Geometry: final body of the model. Coordinates: model frame, mm. A direction names the side the tool comes from. Give positions to 0.01 mm unless a question says otherwise; leave off trailing zeros. Write each loop counter-clockwise with the first axis right and the second up, starting at its lowest first coordinate (ties: lowest second). Pieces come first, ordered by that corner, then holes. Notation, with made-up numbers: (23.25, -2) - (48.25, -2) arc R18 ccw to (48.25, 21) - close; hole circle Ø4 at (75, 24). An arc over 180 degrees is marked (long way). One line per question, with ' | ' between items. Start each with the question number.
```python
from build123d import *

# Parameters (mm, degrees)
SKETCH1_R           = 13
BOSS_EXTRUDE1_DEPTH = 12.5
CUT_EXTRUDE1_START  = 3
SKETCH2_R           = 16
CUT_EXTRUDE1_DEPTH  = 37.563240514
SKETCH3_R           = 2.5
CUT_EXTRUDE2_DEPTH  = 52.285962992
CUT_EXTRUDE3_START  = 10
SKETCH5_R           = 16.85
SKETCH5_R_2         = 16
CUT_EXTRUDE3_DEPTH  = 1.3
CHAMFER2_SIZE       = 0.5


with BuildPart() as part:
    # Sketch1 → Boss-Extrude1 (new body)
    with BuildSketch(Plane.XY):
        with BuildLine():
            Line((25, -28), (-25, -28))
            Line((-25, -28), (-25, -23))
            Line((-25, -23), (-10.297842021, -23))
            Line((-10.297842021, -23), (-10.297842021, -17.145099875))
            ThreePointArc((-10.297842021, -17.145099875), (0, 20), (10.297842021, -17.145099875))
            Line((10.297842021, -17.145099875), (10.297842021, -23))
            Line((10.297842021, -23), (25, -23))
            Line((25, -23), (25, -28))
        make_face()
        Circle(SKETCH1_R, mode=Mode.SUBTRACT)
    extrude(amount=BOSS_EXTRUDE1_DEPTH)

    # Sketch2 → Cut-Extrude1 (cut, through all)
    with BuildSketch(Plane.XY.offset(CUT_EXTRUDE1_START)):
        Circle(SKETCH2_R)
    extrude(amount=CUT_EXTRUDE1_DEPTH, mode=Mode.SUBTRACT)

    # Sketch3 → Cut-Extrude2 (cut, through all)
    with BuildSketch(Plane(origin=(0, -23, 0), x_dir=(1, 0, 0), z_dir=(0, 1, 0))):
        with Locations(Location((-20, -6.25, 0), (0, 0, 180))):
            Circle(SKETCH3_R)
        with Locations(Location((20, -6.25, 0), (0, 0, 180))):
            Circle(SKETCH3_R)
    extrude(amount=-CUT_EXTRUDE2_DEPTH, mode=Mode.SUBTRACT)

    # Sketch5 → Cut-Extrude3 (cut)
    with BuildSketch(Plane.XY.offset(CUT_EXTRUDE3_START)):
        Circle(SKETCH5_R)
        Circle(SKETCH5_R_2, mode=Mode.SUBTRACT)
    extrude(amount=CUT_EXTRUDE3_DEPTH, mode=Mode.SUBTRACT)

    # Chamfer2
    chamfer2_edges = [part.edges().sort_by_distance(p)[0] for p in [
        (-16, 0, 12.5),
    ]]
    chamfer(chamfer2_edges, length=CHAMFER2_SIZE)


solid = part.part
```
1) Pull-direction query (Y, two-part tool) for faces 4 (the flat face through (0, -28, 6)), 5 (the flat face through (-17.75, -23, 4.77)), 6 (the cylindrical face through (-17.502, -25.465, 6.36)); classes: +Y half, -Y half, draft (parallel to the pull), parting line (faces both ways), or undercut.
2) Section A-A, the plane z = 6.25. Output: boundary loops of the cut face in (x, y).
3) Reachability of faces 1 (the flat face through (15, -6, 11.3)), 2 (the flat face through (10.298, -20, 6)), 3 (the flat face through (-10.298, -20, 6)) from +Z, -Z, +X, -X, +Y, -Y: full face, straight path, thin tool, end or side. Return the list, or none.
4) Line query: L1, parallel to Z at x = 20, y = -26.2; L2, parallel to X at y = -24.5, z = 7; L3, parallel to Y at x = 12, z = 9. Output: solid intervals per line, ascending.
5) First-contact query: pin 1 Ø3 at (y, z) = (12.5, 9.5) entering from +X; pin 2 Ø4.5 at (y, z) = (-20.5, 8) entering from +X; pin 3 Ø6 at (x, z) = (19.5, 7.5) entering from +Y. Flat tips, straight axial feed; report the tip coordinate or a pass-through.
6) Section B-B, the plane x = 0. Output: boundary loops of the cut face in (y, z), plus the area to 3 significant figures.
Answer key:
1) face 4: -Y half | face 5: undercut | face 6: draft
2) outline: (-25, -28) - (-22.5, -28) - (-22.5, -23) - (-25, -23) - close; (-17.5, -28) - (17.5, -28) - (17.5, -23) - (10.3, -23) - (10.3, -17.15) arc R20 ccw (long way) to (-10.3, -17.15) - (-10.3, -23) - (-17.5, -23) - close; (22.5, -28) - (25, -28) - (25, -23) - (22.5, -23) - close; hole circle Ø32 at (0, 0)
3) face 1: none | face 2: +Z, -Z, +X | face 3: +Z, -Z, -X
4) L1: 0 to 3.75, 8.75 to 12.5 | L2: -25 to -22.38, -17.62 to 17.62, 22.38 to 25 | L3: -28 to -23, -16 to -10.58, 10.58 to 16
5) pin 1: x = 16.7 | pin 2: x = 10.3 | pin 3: y = 11.3
6) outline: (-28, 0) - (-13, 0) - (-13, 3) - (-16, 3) - (-16, 10) - (-16.85, 10) - (-16.85, 11.3) - (-16, 11.3) - (-16, 12) - (-16.5, 12.5) - (-28, 12.5) - close; (13, 0) - (20, 0) - (20, 12.5) - (16.5, 12.5) - (16, 12) - (16, 11.3) - (16.85, 11.3) - (16.85, 10) - (16, 10) - (16, 3) - (13, 3) - close | area: 216 mm^2
